Can you work these out from the model? Positions are in its coordinate system, mm. A direction names the side the tool comes from. Coordinates: 2 decimals unless noted, no trailing zeros. Order: outer loops, then holes, each group sorted by start corner. A loop starts at its lowest first (then second) coordinate and runs counter-clockwise, first axis right, second up.
```python
from build123d import *

# Parameters (mm, degrees)
EXTRUDE_1_DEPTH          = 30
CUT_EXTRUDE_1_DEPTH      = 65.652919501
CUT_EXTRUDE_1_DEPTH_BACK = 65.652919501
EXTRUDE_2_DEPTH          = 8
EXTRUDE_3_DEPTH          = 4


with BuildPart() as part:
    # 草图1 → 凸台-拉伸1 (new body)
    with BuildSketch(Plane(origin=(0, 0, 0), x_dir=(1, 0, 0), z_dir=(0, 1, 0))):
        Polygon((0, 0), (56, 0), (56, 8), (32, 8), (32, 12), (0, 12), align=None)
    extrude(amount=EXTRUDE_1_DEPTH)

    # 草图2 → 切除-拉伸1 (cut, two sides: drawn at the far end of the back side and taken through both)
    with BuildSketch(Plane.ZY.offset(-CUT_EXTRUDE_1_DEPTH_BACK)):
        Polygon((0, 15), (0, 15.000747226), (0, 21), (-5, 23.886751346), (-5, 6.11399588), (0, 9.000747226), align=None)
    extrude(amount=CUT_EXTRUDE_1_DEPTH + CUT_EXTRUDE_1_DEPTH_BACK, mode=Mode.SUBTRACT)

    # 草图5 → 凸台-拉伸2 (add)
    with BuildSketch(Plane.XZ):
        with BuildLine():
            Line((56, -8), (44, -8))
            Line((44, -8), (32, -8))
            Line((32, -8), (32, -12))
            Line((32, -12), (0, -12))
            Line((0, -12), (0, -20))
            Line((0, -20), (40.466636051, -32.468013743))
            ThreePointArc((40.466636051, -32.468013743), (51.127398986, -30.654024223), (56, -21))
            Line((56, -21), (56, -8))
        make_face()
        with BuildLine():
            ThreePointArc((38, -16), (39.757359313, -11.757359313), (44, -10))
            ThreePointArc((44, -10), (48.242640687, -11.757359313), (50, -16))
            Line((50, -16), (50, -21))
            ThreePointArc((50, -21), (44, -27), (38, -21))
            Line((38, -21), (38, -16))
        make_face(mode=Mode.SUBTRACT)
    extrude(amount=-EXTRUDE_2_DEPTH)

    # 草图6 → 凸台-拉伸3 (add)
    with BuildSketch(Plane(origin=(0, 8, 0), x_dir=(1, 0, 0), z_dir=(0, 1, 0))):
        with BuildLine():
            Line((32, 21), (32, 8))
            Line((32, 8), (56, 8))
            Line((56, 8), (56, 21))
            ThreePointArc((56, 21), (44, 33), (32, 21))
        make_face()
        with BuildLine():
            Line((38, 21), (38, 16))
            ThreePointArc((38, 16), (44, 10), (50, 16))
            Line((50, 16), (50, 21))
            ThreePointArc((50, 21), (44, 27), (38, 21))
        make_face(mode=Mode.SUBTRACT)
    extrude(amount=EXTRUDE_3_DEPTH)


solid = part.part
```
1. Imagine slicing it at A-A on y = 18.5. Please give me the cut outline in (x, z).
Completed:
outline: (0, -12) - (32, -12) - (32, -8) - (56, -8) - (56, -5) - (0, -5) - close
2. Imagine slicing it at D-D on x = 47.5. Please give me the cut outline in (y, z).
Completed:
outline: (0, -32.48) - (12, -32.48) - (12, -25.87) - (0, -25.87) - close; (0, -11.13) - (12, -11.13) - (12, -8) - (30, -8) - (30, 0) - (21, 0) - (23.89, -5) - (6.11, -5) - (9, 0) - (0, 0) - close
3. Thinking about a two-plate mould opening in X: for faces 1 (the flat face through (44, 21, -8)), 2 (the flat face through (38, 6, -19)), 3 (the flat face through (56, 11, -10)), which applies, pulls with the +X half, pulls with the -X half, needs draft (parallel to the pull), parting line crosses it, or undercut?
Completed:
face 1: needs draft
face 2: undercut
face 3: pulls with the +X half
4. Please list where these lines run through material, in increasing order: probe 1 along Z at (x, y) = (44, 6.75); probe 2 along Y at (x, z) = (23, -19.5); probe 3 along Z at (x, y) = (12, 10).
Completed:
probe 1: z = -33 to -27, -10 to -5, -3.9 to 0
probe 2: y = 0 to 8
probe 3: z = -12 to -5
5. On a 3-axis mill with a long thin cutter (end or side, diameter ignored), from which of +Z, -Z, +X, -X, +Y, -Y can I reach the whole of each face in a straight line? I mean faces 4 (the cylindrical face through (48.351, 7.249, -32.183)), 5 (the flat face through (20, 8, -20)), 6 (the flat face through (32, 21, -10)), 7 (the cylindrical face through (44, 6, -27)). Say none if no direction works.
Completed:
face 4: -Z, +Y
face 5: -Z, -X, +Y
face 6: -Z, +X, +Y
face 7: +Y, -Y
6. Imagine slicing it at C-C on x = 30. Please give me the cut outline in (y, z).
Completed:
outline: (0, -29.24) - (8, -29.24) - (8, -12) - (30, -12) - (30, 0) - (21, 0) - (23.89, -5) - (6.11, -5) - (9, 0) - (0, 0) - close
7. Imagine slicing it at B-B on z = -22. Please give me the cut outline in (x, y), then the cut area to 3 significant figures.
Completed:
outline: (6.49, 0) - (38.08, 0) - (38.08, 12) - (32.04, 12) - (32.04, 8) - (6.49, 8) - close; (49.92, 0) - (55.96, 0) - (55.96, 12) - (49.92, 12) - close
area: 349 mm2
8. I'm going to push flat-ended pins straight in: pin 1 (14.5 mm diameter, centred on x = 48.5, y = 19, fed in from -Z); pin 2 (8 mm diameter, centred on x = 32.5, y = 18, fed in from +Z); pin 3 (3 mm diameter, centred on y = 11, z = -17, fed in from -X); pin 4 (10 mm diameter, centred on x = 26, z = -27, fed in from +Y). Where does each tip first touch, or does it pass through?
Completed:
pin 1: stops at z = -32.71
pin 2: stops at z = 0
pin 3: stops at x = 32
pin 4: stops at y = 8
